from build123d import *

# Parameters (mm, degrees)
SKETCH1_R           = 2.5
SKETCH1_R_2         = 20
BOSS_EXTRUDE1_DEPTH = 6.35
FILLET1_R           = 5
FILLET2_R           = 3


with BuildPart() as part:
    # Sketch1 → Boss-Extrude1 (new body)
    with BuildSketch(Plane.XY):
        Polygon((20, 61.824817518), (-60, 61.824817518), (-140, -58.175182482), (-140, -78.175182482), (20, -78.175182482), align=None)
        with Locations((-50, -48.175182482)):
            Circle(SKETCH1_R, mode=Mode.SUBTRACT)
        with Locations((-50, -28.175182482)):
            Circle(SKETCH1_R, mode=Mode.SUBTRACT)
        with Locations((-50, -8.175182482)):
            Circle(SKETCH1_R, mode=Mode.SUBTRACT)
        with Locations((-50, 11.824817518)):
            Circle(SKETCH1_R, mode=Mode.SUBTRACT)
        with Locations((-50, 31.824817518)):
            Circle(SKETCH1_R, mode=Mode.SUBTRACT)
        with Locations((-50, 51.824817518)):
            Circle(SKETCH1_R, mode=Mode.SUBTRACT)
        with Locations((-30, -48.175182482)):
            Circle(SKETCH1_R, mode=Mode.SUBTRACT)
        with Locations((-30, 51.824817518)):
            Circle(SKETCH1_R, mode=Mode.SUBTRACT)
        with Locations((-10, 1.824817518)):
            Circle(SKETCH1_R_2, mode=Mode.SUBTRACT)
        with Locations((-30, -68.175182482)):
            Circle(SKETCH1_R, mode=Mode.SUBTRACT)
        with Locations((-50, -68.175182482)):
            Circle(SKETCH1_R, mode=Mode.SUBTRACT)
        with Locations((-70, -68.175182482)):
            Circle(SKETCH1_R, mode=Mode.SUBTRACT)
        with Locations((-90, -68.175182482)):
            Circle(SKETCH1_R, mode=Mode.SUBTRACT)
        with Locations((-110, -68.175182482)):
            Circle(SKETCH1_R, mode=Mode.SUBTRACT)
        with Locations((-130, -68.175182482)):
            Circle(SKETCH1_R, mode=Mode.SUBTRACT)
        with Locations((-33.5, 25.324817518)):
            Circle(SKETCH1_R, mode=Mode.SUBTRACT)
        with Locations((13.5, 25.324817518)):
            Circle(SKETCH1_R, mode=Mode.SUBTRACT)
        with Locations((13.5, -21.675182482)):
            Circle(SKETCH1_R, mode=Mode.SUBTRACT)
        with Locations((-33.5, -21.675182482)):
            Circle(SKETCH1_R, mode=Mode.SUBTRACT)
    extrude(amount=BOSS_EXTRUDE1_DEPTH)

    # Fillet1
    fillet1_edges = [part.edges().sort_by_distance(p)[0] for p in [
        (-140, -58.175182482, 3.175),
        (-60, 61.824817518, 3.175),
    ]]
    fillet(fillet1_edges, radius=FILLET1_R)

    # Fillet2
    fillet2_edges = [part.edges().sort_by_distance(p)[0] for p in [
        (20, -78.175182482, 3.175),
        (-140, -78.175182482, 3.175),
        (20, 61.824817518, 3.175),
    ]]
    fillet(fillet2_edges, radius=FILLET2_R)


solid = part.part
Model file for the job. Use its own axes, mm. Give positions to 0.01 mm unless a question says otherwise; leave off trailing zeros. Loops run counter-clockwise (first coordinate to the right, second up) from the corner with the lowest first, then second, coordinate; pieces in that order, holes last.
1) Flat gauge pins, fed straight in: pin 1 Ø4.5 at (x, y) = (-50, -68.18) entering from -Z; pin 2 Ø8 at (x, y) = (-30, -68.18) entering from -Z; pin 3 Ø1.5 at (y, z) = (-13.5, 2.5) entering from -X. Where does each tip first touch, or does it go through?
2) Wall check: line 1 (Y direction, x = -11, z = 3); line 2 (Y direction, x = -10, z = 3); line 3 (X direction, y = 53.5, z = 4.75). Give the ranges that are in metal, low to high.
3) Saw through at A-A (x = 13.5). Write the cut outline in (y, z), plus the area to 4 significant figures.
4) Pull direction X, two halves, no side cores. Call faces 1 (the cylindrical face through (-48.656, -46.067, 3.131)), 2 (the flat face through (-99.779, 2.157, 3.131)), 3 (the flat face through (20, -9, 3)): +X half, -X half, draft (parallel to the pull), parting line (faces both ways), or undercut.
5) Saw through at C-C (x = -50). Count the separate pieces of the cut face and the enclosed holes in it, plus the area to 3 significant figures.
6) Saw through at B-B (x = -10). Write the cut outline in (y, z), plus the area to 3 significant figures.
Answer block:
1. pin 1: passes through
1. pin 2: stops at z = 0
1. pin 3: stops at x = -110.72
2. line 1: y = -78.18 to -18.15, 21.8 to 61.82
2. line 2: y = -78.18 to -18.18, 21.82 to 61.82
2. line 3: x = -65.55 to -51.86, -48.14 to -31.86, -28.14 to 20
3. outline: (-78.18, 0) - (-24.18, 0) - (-24.18, 6.35) - (-78.18, 6.35) - close; (-19.18, 0) - (22.82, 0) - (22.82, 6.35) - (-19.18, 6.35) - close; (27.82, 0) - (61.82, 0) - (61.82, 6.35) - (27.82, 6.35) - close
3. area: 825.5 mm2
4. face 1: undercut
4. face 2: -X half
4. face 3: +X half
5. separate pieces: 8
5. enclosed holes: 0
5. area: 667 mm2
6. outline: (-78.18, 0) - (-18.18, 0) - (-18.18, 6.35) - (-78.18, 6.35) - close; (21.82, 0) - (61.82, 0) - (61.82, 6.35) - (21.82, 6.35) - close
6. area: 635 mm2
